For this review, use the dimensioned drawing (mm, ordinates from the lowest corner) and the shaded views. A direction names the side the tool comes from. Round coordinates to 2 decimals unless told otherwise and drop trailing zeros. Order: outer loops, then holes, each group sorted by start corner. A loop starts at its lowest first (then second) coordinate and runs counter-clockwise, first axis right, second up. Notation, with made-up numbers: (-25.5, 84.5) -> (23.5, 84.5) arc R24 ccw to (23.5, 98.5) -> close; hole circle Ø8 at (-10, 51.25). An arc over 180 degrees is marked (long way). Answer in a Markdown table with one row per item.
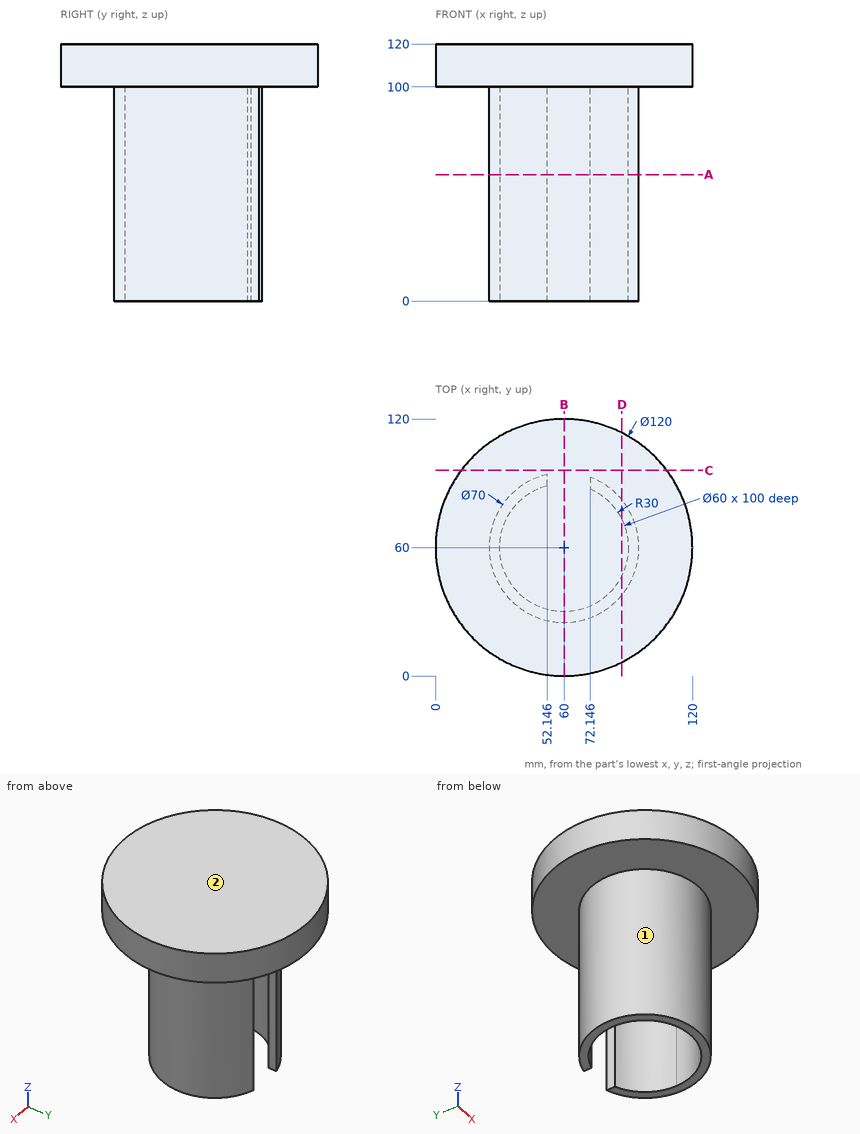
Q1. Clearance check with flat-ended pins moving along their axes: pin 1 Ø4 at (x, z) = (29, 50) entering from -Y (1 decimal); pin 2 Ø2.5 at (y, z) = (90.5, 37.5) entering from -X; pin 3 Ø10 at (x, y) = (73.5, 69.5) entering from -Z. State where each tip first meets the part, or that it passes through.
Answer key:
| item | result |
|---|---|
| pin 1 | stops at y = 40.4 |
| pin 2 | stops at x = 40.78 |
| pin 3 | stops at z = 100 |
Q2. Take a section at C-C, the plane y = 96. Write out the cut boundary in (x, z).
Answer key:
| item | result |
|---|---|
| outline | (12, 100) -> (108, 100) -> (108, 120) -> (12, 120) -> close |
Q3. Take a section at D-D, the plane x = 87. Write out the cut boundary in (y, z).
Answer key:
| item | result |
|---|---|
| outline | (6.42, 100) -> (37.73, 100) -> (37.73, 0) -> (46.92, 0) -> (46.92, 100) -> (73.08, 100) -> (73.08, 0) -> (82.27, 0) -> (82.27, 100) -> (113.58, 100) -> (113.58, 120) -> (6.42, 120) -> close |
Q4. Take a section at A-A, the plane z = 59. Write out the cut boundary in (x, y) (1 decimal), then the cut area to 3 significant figures.
Answer key:
| item | result |
|---|---|
| outline | (52.1, 89) -> (52.1, 94.1) arc R35 ccw (long way) to (72.1, 92.8) -> (72.1, 87.4) arc R30 cw (long way) to start |
| area | 919 mm^2 |
Q5. To check wall thickness, follow probe 1 along X at (y, z) = (60, 57); probe 2 along Z at (x, y) = (67.5, 34.5); probe 3 along Y at (x, z) = (60, 79.5). State the ranges of each line that lie inside material, in increasing order.
Answer key:
| item | result |
|---|---|
| probe 1 | x = 25 to 30, 90 to 95 |
| probe 2 | z = 100 to 120 |
| probe 3 | y = 25 to 30 |
Q6. Tool access review of the marked faces 1 and 2: name each direction out of +Z, -Z, +X, -X, +Y, -Y from which nothing blocks a thin tool from reaching the whole face with its end or side.
Answer key:
| item | result |
|---|---|
| face 1 | -Z |
| face 2 | +Z, +X, -X, +Y, -Y |
Q7. Take a section at B-B, the plane x = 60. Write out the cut boundary in (y, z).
Answer key:
| item | result |
|---|---|
| outline | (0, 100) -> (25, 100) -> (25, 0) -> (30, 0) -> (30, 100) -> (120, 100) -> (120, 120) -> (0, 120) -> close |
